```python
from build123d import *
from build123d.topology import SkipClean

# Parameters (mm, degrees)
EXTRUDE_1_DEPTH       = 1.65
HOLE_WIZARD_M21_D     = 2.4
HOLE_WIZARD_M21_DEPTH = 10
HOLE_WIZARD_M21_TIP   = 0.721032743
SKETCH_5_R            = 0.45
CUT_EXTRUDE_1_DEPTH   = 35.039609281
EXTRUDE_2_DEPTH       = 0.1
EXTRUDE_2_DEPTH_BACK  = 1.75
SKETCH_6_R            = 2
SKETCH_6_R_2          = 1.2
SKETCH_6_R_3          = 0.75
SKETCH_6_R_4          = 0.45
SKETCH_7_W            = 2.5
SKETCH_7_H            = 0.9
SKETCH_7_W_2          = 3.5
SKETCH_7_H_2          = 1.8
EXTRUDE_3_DEPTH       = 0.1


with BuildPart() as part:
    # Эскиз1 → Бобышка-Вытянуть1 (new body)
    with BuildSketch(Plane.XY):
        with BuildLine():
            Line((-27.15, -17.5), (27.15, -17.5))
            ThreePointArc((27.15, -17.5), (28.564213562, -16.914213562), (29.15, -15.5))
            Line((29.15, -15.5), (29.15, 15.5))
            ThreePointArc((29.15, 15.5), (28.564213562, 16.914213562), (27.15, 17.5))
            Line((27.15, 17.5), (-27.15, 17.5))
            ThreePointArc((-27.15, 17.5), (-28.564213562, 16.914213562), (-29.15, 15.5))
            Line((-29.15, 15.5), (-29.15, -15.5))
            ThreePointArc((-29.15, -15.5), (-28.564213562, -16.914213562), (-27.15, -17.5))
        make_face()
    extrude(amount=EXTRUDE_1_DEPTH)

    # Отверстие с зазором M21
    with Locations(Plane.XY.offset(1.65)):
        with Locations((26.65, 15), (-26.65, -15), (-26.65, 15), (26.65, -15)):
            Hole(HOLE_WIZARD_M21_D / 2, depth=HOLE_WIZARD_M21_DEPTH)
            with Locations((0, 0, -(HOLE_WIZARD_M21_DEPTH + HOLE_WIZARD_M21_TIP / 2))):  # 118° drill point
                Cone(0, HOLE_WIZARD_M21_D / 2, HOLE_WIZARD_M21_TIP, mode=Mode.SUBTRACT)

    # Эскиз5 → Вырез-Вытянуть1 (cut, through all)
    with BuildSketch(Plane.XY.offset(1.65)):
        with Locations((26.65, -8.89)):
            Circle(SKETCH_5_R)
        with Locations((26.65, -6.35)):
            Circle(SKETCH_5_R)
        with Locations((26.65, -3.81)):
            Circle(SKETCH_5_R)
        with Locations((26.65, -1.27)):
            Circle(SKETCH_5_R)
        with Locations((26.65, 1.27)):
            Circle(SKETCH_5_R)
        with Locations((26.65, 3.81)):
            Circle(SKETCH_5_R)
        with Locations((26.65, 6.35)):
            Circle(SKETCH_5_R)
        with Locations((26.65, 8.89)):
            Circle(SKETCH_5_R)
    extrude(amount=-CUT_EXTRUDE_1_DEPTH, mode=Mode.SUBTRACT)

    # Эскиз6 → Бобышка-Вытянуть2 (add, two sides: drawn at the far end of the back side and taken through both)
    # profile 1 of 12: a face of its own
    with SkipClean():  # the faces are left unmerged after this step: merging them gives an invalid solid
        with BuildSketch(Plane.XY.offset(1.65).offset(-EXTRUDE_2_DEPTH_BACK)):
            with Locations(Location((-26.65, 15, 0), (0, 0, 180))):
                Circle(SKETCH_6_R)
            with Locations((-26.65, 15)):
                Circle(SKETCH_6_R_2, mode=Mode.SUBTRACT)
        # profile 2 of 12: a face of its own
        with BuildSketch(Plane.XY.offset(1.65).offset(-EXTRUDE_2_DEPTH_BACK)):
            with Locations(Location((26.65, 15, 0), (0, 0, 180))):
                Circle(SKETCH_6_R)
            with Locations((26.65, 15)):
                Circle(SKETCH_6_R_2, mode=Mode.SUBTRACT)
        # profile 3 of 12: a face of its own
        with BuildSketch(Plane.XY.offset(1.65).offset(-EXTRUDE_2_DEPTH_BACK)):
            with Locations(Location((26.65, -15, 0), (0, 0, 180))):
                Circle(SKETCH_6_R)
            with Locations((26.65, -15)):
                Circle(SKETCH_6_R_2, mode=Mode.SUBTRACT)
        # profile 4 of 12: a face of its own
        with BuildSketch(Plane.XY.offset(1.65).offset(-EXTRUDE_2_DEPTH_BACK)):
            with Locations(Location((-26.65, -15, 0), (0, 0, 180))):
                Circle(SKETCH_6_R)
            with Locations((-26.65, -15)):
                Circle(SKETCH_6_R_2, mode=Mode.SUBTRACT)
        # profile 5 of 12: a face of its own
        with BuildSketch(Plane.XY.offset(1.65).offset(-EXTRUDE_2_DEPTH_BACK)):
            with Locations(Location((26.65, -8.89, 0), (0, 0, 180))):
                Circle(SKETCH_6_R_3)
            with Locations((26.65, -8.89)):
                Circle(SKETCH_6_R_4, mode=Mode.SUBTRACT)
        # profile 6 of 12: a face of its own
        with BuildSketch(Plane.XY.offset(1.65).offset(-EXTRUDE_2_DEPTH_BACK)):
            with Locations(Location((26.65, -6.35, 0), (0, 0, 180))):
                Circle(SKETCH_6_R_3)
            with Locations((26.65, -6.35)):
                Circle(SKETCH_6_R_4, mode=Mode.SUBTRACT)
        # profile 7 of 12: a face of its own
        with BuildSketch(Plane.XY.offset(1.65).offset(-EXTRUDE_2_DEPTH_BACK)):
            with Locations(Location((26.65, -3.81, 0), (0, 0, 180))):
                Circle(SKETCH_6_R_3)
            with Locations((26.65, -3.81)):
                Circle(SKETCH_6_R_4, mode=Mode.SUBTRACT)
        # profile 8 of 12: a face of its own
        with BuildSketch(Plane.XY.offset(1.65).offset(-EXTRUDE_2_DEPTH_BACK)):
            with Locations(Location((26.65, -1.27, 0), (0, 0, 180))):
                Circle(SKETCH_6_R_3)
            with Locations((26.65, -1.27)):
                Circle(SKETCH_6_R_4, mode=Mode.SUBTRACT)
        # profile 9 of 12: a face of its own
        with BuildSketch(Plane.XY.offset(1.65).offset(-EXTRUDE_2_DEPTH_BACK)):
            with Locations(Location((26.65, 1.27, 0), (0, 0, 180))):
                Circle(SKETCH_6_R_3)
            with Locations((26.65, 1.27)):
                Circle(SKETCH_6_R_4, mode=Mode.SUBTRACT)
        # profile 10 of 12: a face of its own
        with BuildSketch(Plane.XY.offset(1.65).offset(-EXTRUDE_2_DEPTH_BACK)):
            with Locations(Location((26.65, 3.81, 0), (0, 0, 180))):
                Circle(SKETCH_6_R_3)
            with Locations((26.65, 3.81)):
                Circle(SKETCH_6_R_4, mode=Mode.SUBTRACT)
        # profile 11 of 12: a face of its own
        with BuildSketch(Plane.XY.offset(1.65).offset(-EXTRUDE_2_DEPTH_BACK)):
            with Locations(Location((26.65, 6.35, 0), (0, 0, 180))):
                Circle(SKETCH_6_R_3)
            with Locations((26.65, 6.35)):
                Circle(SKETCH_6_R_4, mode=Mode.SUBTRACT)
        # profile 12 of 12: a face of its own
        with BuildSketch(Plane.XY.offset(1.65).offset(-EXTRUDE_2_DEPTH_BACK)):
            with Locations(Location((26.65, 8.89, 0), (0, 0, 180))):
                Circle(SKETCH_6_R_3)
            with Locations((26.65, 8.89)):
                Circle(SKETCH_6_R_4, mode=Mode.SUBTRACT)
        extrude(amount=EXTRUDE_2_DEPTH + EXTRUDE_2_DEPTH_BACK)
    add(part.part.scale(1), mode=Mode.REPLACE)  # the faces are merged on a copy

    # Эскиз7 → Бобышка-Вытянуть3 (add)
    with BuildSketch(Plane(origin=(0, 0, 0), x_dir=(-1, 0, 0), z_dir=(0, 0, -1))):
        with Locations((17.2, -5)):
            Rectangle(SKETCH_7_W, SKETCH_7_H)
        with Locations((17.2, -7)):
            Rectangle(SKETCH_7_W, SKETCH_7_H)
        with Locations((17.2, -3)):
            Rectangle(SKETCH_7_W, SKETCH_7_H)
        with Locations((17.2, -1)):
            Rectangle(SKETCH_7_W, SKETCH_7_H)
        with Locations((17.2, 1)):
            Rectangle(SKETCH_7_W, SKETCH_7_H)
        with Locations((17.2, 3)):
            Rectangle(SKETCH_7_W, SKETCH_7_H)
        with Locations((17.2, 5)):
            Rectangle(SKETCH_7_W, SKETCH_7_H)
        with Locations((17.2, 7)):
            Rectangle(SKETCH_7_W, SKETCH_7_H)
        with Locations((23.2, -9.65)):
            Rectangle(SKETCH_7_W_2, SKETCH_7_H_2)
        with Locations((23.2, 9.65)):
            Rectangle(SKETCH_7_W_2, SKETCH_7_H_2)
    extrude(amount=EXTRUDE_3_DEPTH)


solid = part.part
```
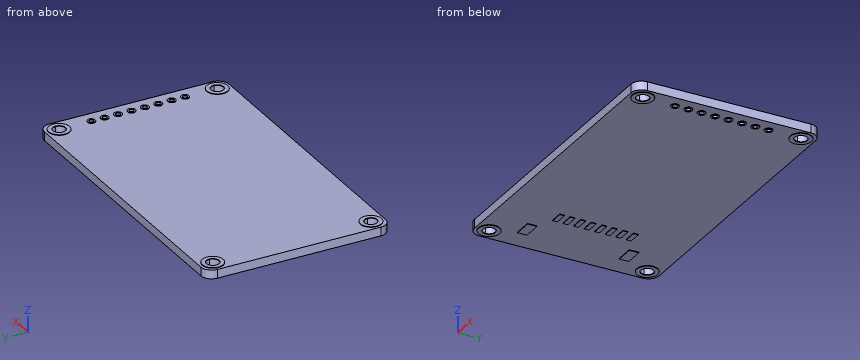
Here's how the part is built. I have some questions about the finished solid (model axes, mm). Coordinates: 2 decimals unless noted, no trailing zeros. Loops run counter-clockwise (first coordinate to the right, second up) from the corner with the lowest first, then second, coordinate; pieces in that order, holes last. Notation, with made-up numbers: (72, 27) - (77, 27) arc R8 ccw to (77, 32) - close; hole circle Ø5 at (11.25, -24.5). An arc over 180 degrees is marked (long way). Return JSON: item names as keys, results as strings. Group by question number.
Item 1: Will these pins go through, and if not, where does the flat tip stop? P1, Ø6, axis at x = 11, y = 8.5, coming from the +Z side; P2, Ø2, axis at x = -26.65, y = -15, coming from the -Z side.
Item 2: If we section it at A-A on x = 8: Write out the boundary of the cut face in (y, z), and give its area (4 significant figures).
Item 3: I need wall thicknesses on line 1 (X direction, y = -15, z = 0.75); line 2 (X direction, y = -15, z = 1.7); line 3 (Y direction, x = -26.65, z = -0.05). Which ranges of each line are inside material? Lowest first, please. Write a range as from..to.
Calculated:
{
 "1": {"P1": "stops at z = 1.65", "P2": "passes through"},
 "2": {"outline": "(-17.5, 0) - (17.5, 0) - (17.5, 1.65) - (-17.5, 1.65) - close", "area": "57.75 mm^2"},
 "3": {"line 1": "x = -29.15..-27.85, -25.45..25.45, 27.85..29.15", "line 2": "x = -28.65..-27.85, -25.45..-24.65, 24.65..25.45, 27.85..28.65", "line 3": "y = -17..-16.2, -13.8..-13, 13..13.8, 16.2..17"}
}
